Verification items for the finished model (mm, model axes). Round coordinates to 2 decimals unless told otherwise and drop trailing zeros. Loops run counter-clockwise (first coordinate to the right, second up) from the corner with the lowest first, then second, coordinate; pieces in that order, holes last.
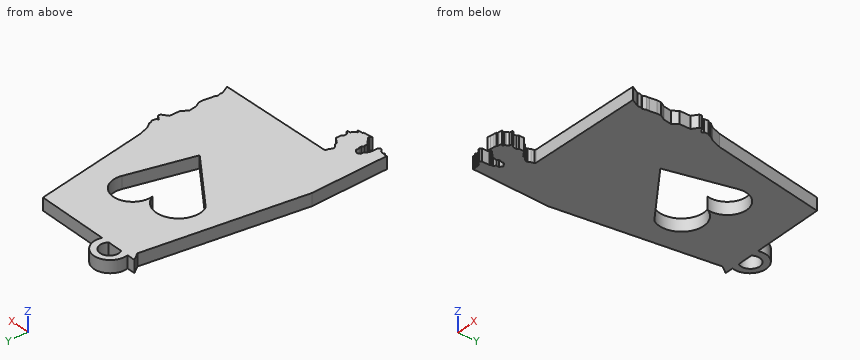
from build123d import *

# Parameters (mm, degrees)
F1_DEPTH = 2.54


with BuildPart() as f1:
    # F0 (on Top) → F1 (new body)
    with BuildSketch(Plane.XY):
        with BuildLine():
            Line((-13.030899, 23.250838), (-14.7814, 23.26861))
            Line((-14.7814, 23.26861), (-13.591297, 21.67334))
            Line((-13.591297, 21.67334), (-17.65191, -11.280064))
            Line((-17.65191, -11.280064), (-16.861185, -27.526684))
            Line((-16.861185, -27.526684), (-16.776092, -27.455773))
            Line((-16.776092, -27.455773), (-16.336445, -27.455773))
            Line((-16.336445, -27.455773), (-16.166259, -27.660001))
            Line((-16.166259, -27.660001), (-15.981892, -27.660001))
            Line((-15.981892, -27.660001), (-15.854253, -27.512502))
            Line((-15.854253, -27.512502), (-15.64152, -27.512502))
            Line((-15.64152, -27.512502), (-15.208855, -27.660001))
            Line((-15.208855, -27.660001), (-14.767447, -28.138192))
            Line((-14.767447, -28.138192), (-14.454785, -28.138192))
            Line((-14.454785, -28.138192), (-14.234081, -27.762407))
            Line((-14.234081, -27.762407), (-14.234081, -26.243819))
            Line((-14.234081, -26.243819), (-14.086945, -26.03608))
            Line((-14.086945, -26.03608), (-14.086945, -25.673669))
            Line((-14.086945, -25.673669), (-13.921417, -25.489749))
            Line((-13.921417, -25.489749), (-13.700713, -25.269045))
            Line((-13.700713, -25.269045), (-13.700713, -24.882814))
            Line((-13.700713, -24.882814), (-13.700713, -24.662109))
            Line((-13.700713, -24.662109), (-13.443226, -24.519552))
            Line((-13.443226, -24.519552), (-13.148954, -24.275878))
            Line((-13.148954, -24.275878), (-12.909858, -24.404623))
            Line((-12.909858, -24.404623), (-12.597195, -24.519552))
            Line((-12.597195, -24.519552), (-12.321316, -24.84603))
            Line((-12.321316, -24.84603), (-12.321316, -25.489749))
            Line((-12.321316, -25.489749), (-12.148302, -25.576962))
            Line((-12.148302, -25.576962), (-12.148302, -26.03608))
            Line((-12.148302, -26.03608), (-12.424181, -26.459094))
            Line((-12.424181, -26.459094), (-12.424181, -26.551055))
            Line((-12.424181, -26.551055), (-12.258654, -26.661407))
            Line((-12.258654, -26.661407), (-12.258654, -27.194774))
            Line((-12.258654, -27.194774), (-11.872422, -27.581004))
            Line((-11.872422, -27.581004), (-10.787295, -28.537387))
            Line((-10.787295, -28.537387), (-10.787295, -28.850051))
            Line((-10.787295, -28.850051), (-11.099959, -29.217891))
            Line((-11.099959, -29.217891), (-10.5482, -29.089147))
            Line((-10.5482, -29.089147), (-9.646993, -29.015578))
            Line((-9.646993, -29.015578), (-9.168802, -28.905228))
            Line((-9.168802, -28.905228), (-9.168802, -28.7397))
            Line((-9.168802, -28.7397), (-8.812965, -28.7397))
            Line((-8.812965, -28.7397), (-8.12046, -28.629348))
            Line((-8.12046, -28.629348), (-8.12046, -28.537387))
            Line((-8.12046, -28.537387), (-8.488759, -28.454099))
            Line((-8.488759, -28.454099), (-8.488759, -28.239436))
            Line((-8.488759, -28.239436), (-8.202543, -28.096328))
            Line((-8.202543, -28.096328), (-8.01173, -27.762407))
            Line((-8.01173, -27.762407), (-7.749365, -27.356932))
            Line((-7.749365, -27.356932), (-7.225457, -27.271397))
            Line((-7.225457, -27.271397), (-7.129228, -27.046863))
            Line((-7.129228, -27.046863), (-7.463148, -26.903754))
            Line((-7.463148, -26.903754), (-7.725514, -26.689092))
            Line((-7.725514, -26.689092), (-7.820919, -26.379023))
            Line((-7.820919, -26.379023), (-7.820919, -25.925847))
            Line((-7.820919, -25.925847), (-7.548839, -25.576962))
            Line((-7.548839, -25.576962), (-7.548839, -24.519552))
            Line((-7.548839, -24.519552), (-8.812965, -23.684751))
            Line((-8.812965, -23.684751), (-8.812965, -23.374682))
            Line((-8.812965, -23.374682), (-9.647765, -22.539882))
            Line((-9.647765, -22.539882), (-9.647765, -22.110555))
            Line((-9.647765, -22.110555), (-9.3854, -21.609675))
            Line((-9.3854, -21.609675), (-9.242291, -20.965688))
            Line((-9.242291, -20.965688), (-9.039888, -20.864896))
            Line((-9.039888, -20.864896), (15.167137, -20.501176))
            Line((15.167137, -20.501176), (14.270123, -18.830877))
            Line((14.270123, -18.830877), (14.270123, -18.181315))
            Line((14.270123, -18.181315), (14.053603, -17.717343))
            Line((14.053603, -17.717343), (14.331986, -17.005919))
            Line((14.331986, -17.005919), (14.331986, -16.387288))
            Line((14.331986, -16.387288), (14.528844, -14.995371))
            Line((14.528844, -14.995371), (14.528844, -14.144757))
            Line((14.528844, -14.144757), (13.852579, -13.000309))
            Line((13.852579, -13.000309), (13.592477, -11.335658))
            Line((13.592477, -11.335658), (14.424803, -10.19121))
            Line((14.424803, -10.19121), (14.424803, -7.902314))
            Line((14.424803, -7.902314), (15.641566, -7.017968))
            Line((15.641566, -7.017968), (15.641566, -6.522429))
            Line((15.641566, -6.522429), (14.685183, -5.915494))
            Line((14.685183, -5.915494), (15.053023, -5.621222))
            Line((15.053023, -5.621222), (15.144982, -4.793584))
            Line((15.144982, -4.793584), (14.8241, -4.396295))
            Line((14.8241, -4.396295), (14.8241, -4.056049))
            Line((14.8241, -4.056049), (14.019881, -2.973447))
            Line((14.019881, -2.973447), (13.283001, -0.933324))
            Line((13.283001, -0.933324), (8.720862, 23.029998))
            Line((8.720862, 23.029998), (-6.454206, 23.184066))
            ThreePointArc((-6.454206, 23.184066), (-9.698639, 27.542757), (-13.030899, 23.250838))
        make_face()
        with BuildLine():
            ThreePointArc((-2.196216, 9.203731), (1.702882, 14.145155), (5.601981, 9.203731))
            Line((5.601981, 9.203731), (2.364994, -4.332762))
            Line((2.364994, -4.332762), (-10.141549, 4.642522))
            ThreePointArc((-10.141549, 4.642522), (-8.599849, 11.157714), (-2.196216, 9.203731))
        make_face(mode=Mode.SUBTRACT)
        with BuildLine():
            ThreePointArc((-11.403755, 23.234318), (-9.755181, 26.28218), (-8.168829, 23.201475))
            Line((-8.168829, 23.201475), (-11.403755, 23.234318))
        make_face(mode=Mode.SUBTRACT)
    extrude(amount=F1_DEPTH)


solid = f1.part
1. Gauge pin test, flat ends, axial feed: P1, Ø0.9, axis at y = -14.5, z = 1.5, coming from the +X side; P2, Ø1.1, axis at y = -8.5, z = 1.5, coming from the +X side; P3, Ø0.5, axis at y = -25, z = 1, coming from the -X side. Record the tip position at first contact, or that the pin passes through.
2. Section check D-D (y = -9). Enter the section's corners in (x, z), then the cut area to 3 significant figures.
3. Section check B-B (y = 12.5). Enter the section's corners in (x, z), then the cut area to 3 significant figures.
4. Section check C-C (z = 0.75). Give the number of separate pieces and of enclosed holes in the cut face, then the cut area to 3 significant figures.
5. Scan lines: L1, parallel to Y at x = -9, z = 0.6; L2, parallel to Y at x = -9.5, z = 1.35; L3, parallel to X at y = -2.5, z = 0.3. Record each from-to range of solid material in increasing order.
6. Section check A-A (x = 1). Enter the section's corners in (y, z), then the cut area to 3 significant figures.
Taken from the geometry:
1. P1: stops at x = 14.53
1. P2: stops at x = 14.42
1. P3: stops at x = -17
2. outline: (-17.37, 0) - (14.42, 0) - (14.42, 2.54) - (-17.37, 2.54) - close
2. area: 80.8 mm2
3. outline: (-14.72, 0) - (-1.54, 0) - (-1.54, 2.54) - (-14.72, 2.54) - close; (4.94, 0) - (10.73, 0) - (10.73, 2.54) - (4.94, 2.54) - close
3. area: 48.2 mm2
4. separate pieces: 1
4. enclosed holes: 2
4. area: 1,140 mm2
5. L1: y = -28.74 to -23.19, -20.86 to 3.82, 10.9 to 23.21, 26.12 to 27.46
5. L2: y = -28.98 to -22.69, -21.83 to 4.18, 10.48 to 23.21, 26.26 to 27.53
5. L3: x = -16.57 to -0.19, 2.8 to 13.85
6. outline: (-20.71, 0) - (-3.35, 0) - (-3.35, 2.54) - (-20.71, 2.54) - close; (14.08, 0) - (23.11, 0) - (23.11, 2.54) - (14.08, 2.54) - close
6. area: 67.0 mm2
